Design review of the part built by this model. Coordinates are the model's own, in mm. Round coordinates to 2 decimals unless told otherwise and drop trailing zeros. Write each loop counter-clockwise with the first axis right and the second up, starting at its lowest first coordinate (ties: lowest second). Pieces come first, ordered by that corner, then holes. Notation, with made-up numbers: (74, 7.5) - (120, 7.5) arc R26 ccw to (120, 42.5) - close; hole circle Ø7 at (-20, -2.75). An arc over 180 degrees is marked (long way). Use one line per item in the form item = value.
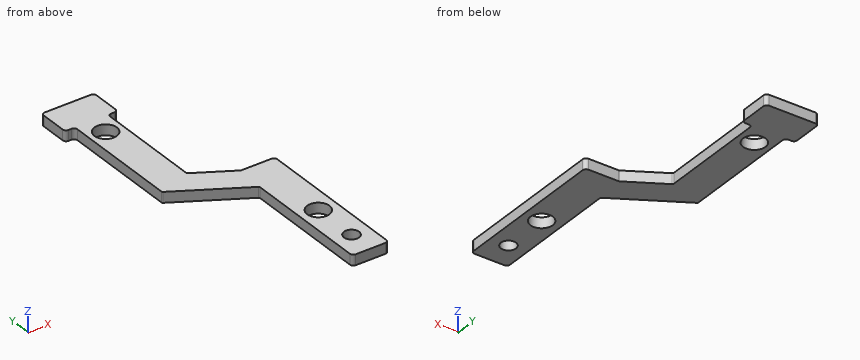
```python
from build123d import *

# Parameters (mm, degrees)
BOARD_DEPTH                  = 1.59144
M3_CLEARANCE_HOLE1_OUTLINE_R = 1.7
M3_CLEARANCE_HOLE1_DEPTH     = 1.59144
SKETCH7_R                    = 1.15
CUTOUT_2_DEPTH               = 53.216689419


# Read off the part's stored shape, not the designer's step: M3 Clearance Hole1
with BuildPart() as part:
    # Sketch1 → Board (new body)
    with BuildSketch(Plane.XY):
        with BuildLine():
            Line((8.00627, 44.00635), (7.50627, 44.00635))
            ThreePointArc((7.50627, 44.00635), (7.152716609, 43.859903391), (7.00627, 43.50635))
            Line((7.00627, 43.50635), (7.00627, 27.50635))
            ThreePointArc((7.00627, 27.50635), (7.039763649, 27.38135), (7.13127, 27.289843649))
            Line((7.13127, 27.289843649), (12.760435125, 24.039843649))
            ThreePointArc((12.760435125, 24.039843649), (12.820730363, 24.014868543), (12.885435125, 24.00635))
            Line((12.885435125, 24.00635), (17.45627, 24.00635))
            ThreePointArc((17.45627, 24.00635), (17.809823391, 23.859903391), (17.95627, 23.50635))
            Line((17.95627, 23.50635), (17.95627, 0.50635))
            ThreePointArc((17.95627, 0.50635), (17.809823391, 0.152796609), (17.45627, 0.00635))
            Line((17.45627, 0.00635), (12.95627, 0.00635))
            ThreePointArc((12.95627, 0.00635), (12.602716609, 0.152796609), (12.45627, 0.50635))
            Line((12.45627, 0.50635), (12.45627, 19.452313745))
            ThreePointArc((12.45627, 19.452313745), (12.422776351, 19.577313745), (12.33127, 19.668820096))
            Line((12.33127, 19.668820096), (2.13127, 25.557792841))
            ThreePointArc((2.13127, 25.557792841), (2.039763649, 25.649299192), (2.00627, 25.774299192))
            Line((2.00627, 25.774299192), (2.00627, 43.50635))
            ThreePointArc((2.00627, 43.50635), (1.859823391, 43.859903391), (1.50627, 44.00635))
            Line((1.50627, 44.00635), (1.00627, 44.00635))
            ThreePointArc((1.00627, 44.00635), (0.652716609, 44.152796609), (0.50627, 44.50635))
            Line((0.50627, 44.50635), (0.50627, 48.50635))
            ThreePointArc((0.50627, 48.50635), (0.652716609, 48.859903391), (1.00627, 49.00635))
            Line((1.00627, 49.00635), (8.00627, 49.00635))
            ThreePointArc((8.00627, 49.00635), (8.359823391, 48.859903391), (8.50627, 48.50635))
            Line((8.50627, 48.50635), (8.50627, 44.50635))
            ThreePointArc((8.50627, 44.50635), (8.359823391, 44.152796609), (8.00627, 44.00635))
        make_face()
    extrude(amount=BOARD_DEPTH)

    # M3 Clearance Hole1 outline → M3 Clearance Hole1 (cut)
    with BuildSketch(Plane.XY):
        with Locations((15.20627, 11.00635)):
            Circle(M3_CLEARANCE_HOLE1_OUTLINE_R)
        with Locations((4.50627, 41.00635)):
            Circle(M3_CLEARANCE_HOLE1_OUTLINE_R)
    extrude(amount=M3_CLEARANCE_HOLE1_DEPTH, mode=Mode.SUBTRACT)

    # Sketch7 → Cutout 2 (cut, through all)
    with BuildSketch(Plane.XY.offset(1.59144)):
        with Locations((15.206, 4.006)):
            Circle(SKETCH7_R)
    extrude(amount=-CUTOUT_2_DEPTH, mode=Mode.SUBTRACT)


solid = part.part
```
Q1. To check wall thickness, follow line 1 along Y through (x, z) = (14.75, 0.2); line 2 along Y through (x, z) = (15, 1.1); line 3 along Y through (x, z) = (17, 0.4). State the ranges of each line that lie inside material, in increasing order. Write a range as from..to.
Calculated:
line_1 = 0.01..2.95, 5.06..9.37, 12.64..24.01
line_2 = 0.01..2.87, 5.14..9.32, 12.69..24.01
line_3 = 0.01..24.01
Q2. We need section C-C on y = 15.5. Write out the cut boundary in (x, z).
Calculated:
outline = (12.46, 0) - (17.96, 0) - (17.96, 1.59) - (12.46, 1.59) - close
Q3. We need section A-A on x = 5. Write out the cut boundary in (y, z).
Calculated:
outline = (23.9, 0) - (39.38, 0) - (39.38, 1.59) - (23.9, 1.59) - close; (42.63, 0) - (49.01, 0) - (49.01, 1.59) - (42.63, 1.59) - close
Q4. We need section D-D on x = 10.75. Write out the cut boundary in (y, z).
Calculated:
outline = (20.58, 0) - (25.2, 0) - (25.2, 1.59) - (20.58, 1.59) - close
Q5. For P1, Ø0.8, axis at x = 16, z = 0.5, coming from the +Y side; P2, Ø0.8, axis at y = 33.5, z = 1, coming from the +X side; P3, Ø2, axis at x = 16, y = 11.5, coming from the -Z side; P4, Ø0.5, axis at y = 7.5, z = 0.5, coming from the -X side, all flat-tipped, find the tip position at first contact; note any pin that passes through.
Calculated:
P1 = 24.01
P2 = 7.01
P3 = 0
P4 = 12.46
Q6. We need section B-B on z = 0.75. State how many separate pieces and enclosed holes the cut face has, then the cut area to 3 significant figures.
Calculated:
separate_pieces = 1
enclosed_holes = 3
area = 274 mm2
